```python
from build123d import *

# Parameters (mm, degrees)
CUT_EXTRUDE1_DEPTH = 28.77920446


with BuildPart() as part:
    # Sketch2 → Revolve1 (revolve)
    with BuildSketch(Plane.XY, mode=Mode.PRIVATE) as revolve1_sk:
        Polygon((0, 9.525), (0, 0), (9.525, 0), (9.525, 10.575392629), (8.881774662, 11.97073299), (8.881774662, 14.296532804), (6.673429623, 14.296532804), (5.487800488, 9.525), align=None)
        Polygon((-9.525, 0), (0, 0), (0, 9.525), (-5.487800488, 9.525), (-6.673429623, 14.296532804), (-8.881774662, 14.296532804), (-8.881774662, 11.97073299), (-9.525, 10.575392629), align=None)
    revolve(revolve1_sk.sketch.rotate(Axis((14.160671305, 0, 0), (-1, 0, 0)), 90), axis=Axis((14.160671305, 0, 0), (-1, 0, 0)))

    # Sketch3 → Cut-Extrude1 (cut, through all)
    with BuildSketch(Plane(origin=(9.525, 0, 0), x_dir=(0, 0, -1), z_dir=(1, 0, 0))):
        Polygon((4.264354564, -5.964781093), (7.297829236, 0.710648837), (3.033474672, 6.67542993), (-4.264354564, 5.964781093), (-7.297829236, -0.710648837), (-3.033474672, -6.67542993), align=None)
    extrude(amount=-CUT_EXTRUDE1_DEPTH, mode=Mode.SUBTRACT)


solid = part.part
```
Model file for the job. Use its own axes, mm. A direction names the side the tool comes from. Coordinates: 2 decimals unless noted, no trailing zeros. Write each loop counter-clockwise with the first axis right and the second up, starting at its lowest first coordinate (ties: lowest second). Pieces come first, ordered by that corner, then holes. Notation, with made-up numbers: (84, 36.5) - (124, 36.5) arc R20 ccw to (124, 40.5) - close; hole circle Ø8 at (83.25, 67). An arc over 180 degrees is marked (long way). One line per item, written item: value. Start each with the question number.
1. Slice it at C-C (y = 0). Write the cut outline in (x, z) (3 decimals).
2. Probe line 1 (Y direction, x = 2, z = 5.5); line 2 (Y direction, x = 8.75, z = -6); line 3 (Z direction, x = -3.25, y = 3). List the from-to ranges inside material, lowest first. Write a range as from..to.
3. Slice it at A-A (x = 8.25). Write the cut outline in (y, z).
4. Slice it at B-B (z = 0). Write the cut outline in (x, y) (3 decimals).
5. Tool access for faces 1 (the flat face through (0.133, -3.651, 5.196)), 2 (the conical face through (-5.56, 9.59, 2.13)), 3 (the flat face through (-8.882, 12, 3)): list every direction of +Z, -Z, +X, -X, +Y, -Y with a clear straight run to the whole face (end or side of a thin tool).
6. Flat gauge pins, fed straight in: pin 1 (6 mm diameter, centred on x = -2.5, y = -11.5, fed in from +Z); pin 2 (4 mm diameter, centred on x = 6.5, y = -3, fed in from +Z); pin 3 (4 mm diameter, centred on x = 3, y = 5.5, fed in from -Z); pin 4 (3 mm diameter, centred on y = 1.5, z = 4.5, fed in from -X). Where does each tip first touch, or does it go through?
7. Slice it at D-D (x = 5). Write the cut outline in (y, z) (3 decimals), plus the area to 3 significant figures.
8. Mould opens along X. For faces 4 (the flat face through (8.882, 12, -3)), 5 (the cylindrical face through (-0.08, 9.3, 2.06)), 6 (the flat face through (0.133, 6.325, 0.564)) say: released by +X, released by -X, zero draft, split by the parting line, or undercut.
Answers below:
1. outline: (-9.525, -10.575) - (-8.882, -11.971) - (-8.882, -14.297) - (-6.673, -14.297) - (-5.488, -9.525) - (5.488, -9.525) - (6.673, -14.297) - (8.882, -14.297) - (8.882, -11.971) - (9.525, -10.575) - (9.525, -6.975) - (-9.525, -6.975) - close; (-9.525, 6.975) - (9.525, 6.975) - (9.525, 10.575) - (8.882, 11.971) - (8.882, 14.297) - (6.673, 14.297) - (5.488, 9.525) - (-5.488, 9.525) - (-6.673, 14.297) - (-8.882, 14.297) - (-8.882, 11.971) - (-9.525, 10.575) - close
2. line 1: y = -7.78..-3.23, 3.25..7.78
2. line 2: y = -12.98..-2.15, 2.53..12.98
2. line 3: z = -9.04..-5.66, 5.61..9.04
3. outline: circle Ø28.59 at (0, 0); hole (-6.68, 3.03) - (-5.96, -4.26) - (0.71, -7.3) - (6.68, -3.03) - (5.96, 4.26) - (-0.71, 7.3) - close
4. outline: (-9.525, -10.575) - (-8.882, -11.971) - (-8.882, -14.297) - (-6.673, -14.297) - (-5.488, -9.525) - (5.488, -9.525) - (6.673, -14.297) - (8.882, -14.297) - (8.882, -11.971) - (9.525, -10.575) - (9.525, -6.38) - (-9.525, -6.38) - close; (-9.525, 6.38) - (9.525, 6.38) - (9.525, 10.575) - (8.882, 11.971) - (8.882, 14.297) - (6.673, 14.297) - (5.488, 9.525) - (-5.488, 9.525) - (-6.673, 14.297) - (-8.882, 14.297) - (-8.882, 11.971) - (-9.525, 10.575) - close
5. face 1: +X, -X
5. face 2: none
5. face 3: -X
6. pin 1: stops at z = 4.3
6. pin 2: stops at z = 14.26
6. pin 3: stops at z = -8.86
6. pin 4: passes through
7. outline: circle Ø19.05 at (0, 0); hole (-6.675, 3.033) - (-5.965, -4.264) - (0.711, -7.298) - (6.675, -3.033) - (5.965, 4.264) - (-0.711, 7.298) - close
7. area: 145 mm^2
8. face 4: released by +X
8. face 5: undercut
8. face 6: zero draft
